```python
from build123d import *

# Parameters (mm, degrees)
F1_DEPTH = 9
F2_DEPTH = 1
F3_START = 8.8
F3_DEPTH = 0.2


with BuildPart() as f1:
    # F0 (on Top) → F1 (new body)
    with BuildSketch(Plane.XY):
        with BuildLine():
            Line((28.9218353152, 47.4191074908), (-98.2781646848, 47.4191074908))
            ThreePointArc((-98.2781646848, 47.4191074908), (-103.2279121531, 45.3688549591), (-105.2781646848, 40.4191074908))
            Line((-105.2781646848, 40.4191074908), (-105.2781646848, -18.9808925092))
            ThreePointArc((-105.2781646848, -18.9808925092), (-103.2279121531, -23.9306399775), (-98.2781646848, -25.9808925092))
            Line((-98.2781646848, -25.9808925092), (28.9218353152, -25.9808925092))
            ThreePointArc((28.9218353152, -25.9808925092), (33.8715827835, -23.9306399775), (35.9218353152, -18.9808925092))
            Line((35.9218353152, -18.9808925092), (35.9218353152, 40.4191074908))
            ThreePointArc((35.9218353152, 40.4191074908), (33.8715827835, 45.3688549591), (28.9218353152, 47.4191074908))
        make_face()
        with BuildLine():
            ThreePointArc((-104.7781646848, 39.9191074908), (-102.7279121531, 44.8688549591), (-97.7781646848, 46.9191074908))
            Line((-97.7781646848, 46.9191074908), (28.4218353152, 46.9191074908))
            ThreePointArc((28.4218353152, 46.9191074908), (33.3715827835, 44.8688549591), (35.4218353152, 39.9191074908))
            Line((35.4218353152, 39.9191074908), (35.4218353152, -18.4808925092))
            ThreePointArc((35.4218353152, -18.4808925092), (33.3715827835, -23.4306399775), (28.4218353152, -25.4808925092))
            Line((28.4218353152, -25.4808925092), (-97.7781646848, -25.4808925092))
            ThreePointArc((-97.7781646848, -25.4808925092), (-102.7279121531, -23.4306399775), (-104.7781646848, -18.4808925092))
            Line((-104.7781646848, -18.4808925092), (-104.7781646848, 10.7191074908))
            Line((-104.7781646848, 10.7191074908), (-104.7781646848, 39.9191074908))
        make_face(mode=Mode.SUBTRACT)
    extrude(amount=F1_DEPTH)

    # F0 (on Top) → F2 (join)
    with BuildSketch(Plane.XY):
        with BuildLine():
            Line((28.9218353152, 47.4191074908), (-98.2781646848, 47.4191074908))
            ThreePointArc((-98.2781646848, 47.4191074908), (-103.2279121531, 45.3688549591), (-105.2781646848, 40.4191074908))
            Line((-105.2781646848, 40.4191074908), (-105.2781646848, -18.9808925092))
            ThreePointArc((-105.2781646848, -18.9808925092), (-103.2279121531, -23.9306399775), (-98.2781646848, -25.9808925092))
            Line((-98.2781646848, -25.9808925092), (28.9218353152, -25.9808925092))
            ThreePointArc((28.9218353152, -25.9808925092), (33.8715827835, -23.9306399775), (35.9218353152, -18.9808925092))
            Line((35.9218353152, -18.9808925092), (35.9218353152, 40.4191074908))
            ThreePointArc((35.9218353152, 40.4191074908), (33.8715827835, 45.3688549591), (28.9218353152, 47.4191074908))
        make_face()
        with BuildLine():
            ThreePointArc((-104.7781646848, 39.9191074908), (-102.7279121531, 44.8688549591), (-97.7781646848, 46.9191074908))
            Line((-97.7781646848, 46.9191074908), (28.4218353152, 46.9191074908))
            ThreePointArc((28.4218353152, 46.9191074908), (33.3715827835, 44.8688549591), (35.4218353152, 39.9191074908))
            Line((35.4218353152, 39.9191074908), (35.4218353152, -18.4808925092))
            ThreePointArc((35.4218353152, -18.4808925092), (33.3715827835, -23.4306399775), (28.4218353152, -25.4808925092))
            Line((28.4218353152, -25.4808925092), (-97.7781646848, -25.4808925092))
            ThreePointArc((-97.7781646848, -25.4808925092), (-102.7279121531, -23.4306399775), (-104.7781646848, -18.4808925092))
            Line((-104.7781646848, -18.4808925092), (-104.7781646848, 10.7191074908))
            Line((-104.7781646848, 10.7191074908), (-104.7781646848, 39.9191074908))
        make_face(mode=Mode.SUBTRACT)
        with BuildLine():
            Line((28.4218353152, 46.9191074908), (-97.7781646848, 46.9191074908))
            ThreePointArc((-97.7781646848, 46.9191074908), (-102.7279121531, 44.8688549591), (-104.7781646848, 39.9191074908))
            Line((-104.7781646848, 39.9191074908), (-104.7781646848, 10.7191074908))
            Line((-104.7781646848, 10.7191074908), (-104.7781646848, -18.4808925092))
            ThreePointArc((-104.7781646848, -18.4808925092), (-102.7279121531, -23.4306399775), (-97.7781646848, -25.4808925092))
            Line((-97.7781646848, -25.4808925092), (28.4218353152, -25.4808925092))
            ThreePointArc((28.4218353152, -25.4808925092), (33.3715827835, -23.4306399775), (35.4218353152, -18.4808925092))
            Line((35.4218353152, -18.4808925092), (35.4218353152, 39.9191074908))
            ThreePointArc((35.4218353152, 39.9191074908), (33.3715827835, 44.8688549591), (28.4218353152, 46.9191074908))
        make_face()
        with BuildLine():
            Line((-104.0281646848, -17.7308925092), (-104.0281646848, 10.7191074908))
            Line((-104.0281646848, 10.7191074908), (-104.0281646848, 39.1691074908))
            ThreePointArc((-104.0281646848, 39.1691074908), (-101.9779121531, 44.1188549591), (-97.0281646848, 46.1691074908))
            Line((-97.0281646848, 46.1691074908), (27.6718353152, 46.1691074908))
            ThreePointArc((27.6718353152, 46.1691074908), (32.6215827835, 44.1188549591), (34.6718353152, 39.1691074908))
            Line((34.6718353152, 39.1691074908), (34.6718353152, -17.7308925092))
            ThreePointArc((34.6718353152, -17.7308925092), (32.6215827835, -22.6806399775), (27.6718353152, -24.7308925092))
            Line((27.6718353152, -24.7308925092), (-97.0281646848, -24.7308925092))
            ThreePointArc((-97.0281646848, -24.7308925092), (-101.9779121531, -22.6806399775), (-104.0281646848, -17.7308925092))
        make_face(mode=Mode.SUBTRACT)
        with BuildLine():
            Line((-104.0281646848, 39.1691074908), (-104.0281646848, 10.7191074908))
            Line((-104.0281646848, 10.7191074908), (-104.0281646848, -17.7308925092))
            ThreePointArc((-104.0281646848, -17.7308925092), (-101.9779121531, -22.6806399775), (-97.0281646848, -24.7308925092))
            Line((-97.0281646848, -24.7308925092), (27.6718353152, -24.7308925092))
            ThreePointArc((27.6718353152, -24.7308925092), (32.6215827835, -22.6806399775), (34.6718353152, -17.7308925092))
            Line((34.6718353152, -17.7308925092), (34.6718353152, 39.1691074908))
            ThreePointArc((34.6718353152, 39.1691074908), (32.6215827835, 44.1188549591), (27.6718353152, 46.1691074908))
            Line((27.6718353152, 46.1691074908), (-97.0281646848, 46.1691074908))
            ThreePointArc((-97.0281646848, 46.1691074908), (-101.9779121531, 44.1188549591), (-104.0281646848, 39.1691074908))
        make_face()
        with BuildLine():
            ThreePointArc((-68.7781646848, 10.7191074908), (-74.5312646848, 4.9660074908), (-80.2843646848, 10.7191074908))
            ThreePointArc((-80.2843646848, 10.7191074908), (-80.2676868415, 11.1568522219), (-80.2177500076, 11.5920589691))
            add(Edge.make_bspline(
                [(-80.2177500076, 11.5920589691), (-79.9166287785, 16.380589161), (-77.2316050473, 21.7170679747), (-74.5312646848, 21.7191074908)],
                knots=[0.0288652727, 0.0288652727, 0.0288652727, 0.0288652727, 0.4998199399, 0.4998199399, 0.4998199399, 0.4998199399], degree=3))
            add(Edge.make_bspline(
                [(-74.5312646848, 21.7191074908), (-71.6633529752, 21.7212735703), (-68.7781646848, 15.7063938677), (-68.7781646848, 10.7191074908)],
                knots=[0.4998199399, 0.4998199399, 0.4998199399, 0.4998199399, 1, 1, 1, 1], degree=3))
        make_face(mode=Mode.SUBTRACT)
        with BuildLine():
            ThreePointArc((28.3885360956, 14.3148952636), (28.6533737253, 14.9542698611), (29.2927483228, 15.2191074908))
            Line((29.2927483228, 15.2191074908), (30.4843238684, 15.2191074908))
            ThreePointArc((30.4843238684, 15.2191074908), (31.1236984659, 14.9542698611), (31.3885360956, 14.3148952636))
            Line((31.3885360956, 14.3148952636), (31.3885360956, 7.1233197179))
            ThreePointArc((31.3885360956, 7.1233197179), (31.1236984659, 6.4839451205), (30.4843238684, 6.2191074908))
            Line((30.4843238684, 6.2191074908), (29.2927483228, 6.2191074908))
            ThreePointArc((29.2927483228, 6.2191074908), (28.6533737253, 6.4839451205), (28.3885360956, 7.1233197179))
            Line((28.3885360956, 7.1233197179), (28.3885360956, 14.3148952636))
        make_face(mode=Mode.SUBTRACT)
    extrude(amount=F2_DEPTH)

    # F0 (on Top) → F3 (join)
    with BuildSketch(Plane.XY.offset(F3_START)):
        with BuildLine():
            Line((28.4218353152, 46.9191074908), (-97.7781646848, 46.9191074908))
            ThreePointArc((-97.7781646848, 46.9191074908), (-102.7279121531, 44.8688549591), (-104.7781646848, 39.9191074908))
            Line((-104.7781646848, 39.9191074908), (-104.7781646848, 10.7191074908))
            Line((-104.7781646848, 10.7191074908), (-104.7781646848, -18.4808925092))
            ThreePointArc((-104.7781646848, -18.4808925092), (-102.7279121531, -23.4306399775), (-97.7781646848, -25.4808925092))
            Line((-97.7781646848, -25.4808925092), (28.4218353152, -25.4808925092))
            ThreePointArc((28.4218353152, -25.4808925092), (33.3715827835, -23.4306399775), (35.4218353152, -18.4808925092))
            Line((35.4218353152, -18.4808925092), (35.4218353152, 39.9191074908))
            ThreePointArc((35.4218353152, 39.9191074908), (33.3715827835, 44.8688549591), (28.4218353152, 46.9191074908))
        make_face()
        with BuildLine():
            Line((-104.0281646848, -17.7308925092), (-104.0281646848, 10.7191074908))
            Line((-104.0281646848, 10.7191074908), (-104.0281646848, 39.1691074908))
            ThreePointArc((-104.0281646848, 39.1691074908), (-101.9779121531, 44.1188549591), (-97.0281646848, 46.1691074908))
            Line((-97.0281646848, 46.1691074908), (27.6718353152, 46.1691074908))
            ThreePointArc((27.6718353152, 46.1691074908), (32.6215827835, 44.1188549591), (34.6718353152, 39.1691074908))
            Line((34.6718353152, 39.1691074908), (34.6718353152, -17.7308925092))
            ThreePointArc((34.6718353152, -17.7308925092), (32.6215827835, -22.6806399775), (27.6718353152, -24.7308925092))
            Line((27.6718353152, -24.7308925092), (-97.0281646848, -24.7308925092))
            ThreePointArc((-97.0281646848, -24.7308925092), (-101.9779121531, -22.6806399775), (-104.0281646848, -17.7308925092))
        make_face(mode=Mode.SUBTRACT)
    extrude(amount=F3_DEPTH)


solid = f1.part
```
Design review of the part built by this model. Coordinates are the model's own, in mm. A direction names the side the tool comes from. Give positions to 0.01 mm unless a question says otherwise; leave off trailing zeros. Write each loop counter-clockwise with the first axis right and the second up, starting at its lowest first coordinate (ties: lowest second). Pieces come first, ordered by that corner, then holes. Notation, with made-up numbers: (51, -1) -> (73, -1) arc R18 ccw to (73, 30) -> close; hole circle Ø4 at (-33, 33). An arc over 180 degrees is marked (long way). Answer in a Markdown table with one row per item.
(1) Consider section C-C (y = 29.5). State the section outline as (x, z) points.
Results:
| item | result |
|---|---|
| outline | (-105.28, 0) -> (35.92, 0) -> (35.92, 9) -> (34.67, 9) -> (34.67, 8.8) -> (35.42, 8.8) -> (35.42, 1) -> (-104.78, 1) -> (-104.78, 8.8) -> (-104.03, 8.8) -> (-104.03, 9) -> (-105.28, 9) -> close |
(2) Consider section A-A (z = 5.75). State the section outline as (x, y) points, then the cut area to 3 significant figures.
Results:
| item | result |
|---|---|
| outline | (-105.28, -18.98) arc R7 ccw to (-98.28, -25.98) -> (28.92, -25.98) arc R7 ccw to (35.92, -18.98) -> (35.92, 40.42) arc R7 ccw to (28.92, 47.42) -> (-98.28, 47.42) arc R7 ccw to (-105.28, 40.42) -> close; hole (-104.78, -18.48) arc R7 ccw to (-97.78, -25.48) -> (28.42, -25.48) arc R7 ccw to (35.42, -18.48) -> (35.42, 39.92) arc R7 ccw to (28.42, 46.92) -> (-97.78, 46.92) arc R7 ccw to (-104.78, 39.92) -> close |
| area | 214 mm2 |
(3) Clearance check with flat-ended pins moving along their axes: pin 1 (12 mm diameter, centred on x = -68.5, y = 21.5, fed in from +Z); pin 2 (0.8 mm diameter, centred on x = 30, z = 0.5, fed in from +Y); pin 3 (1.1 mm diameter, centred on x = 30, z = 0.5, fed in from -Y). State where each tip first meets the part, or that it passes through.
Results:
| item | result |
|---|---|
| pin 1 | z = 1 |
| pin 2 | y = 47.39 |
| pin 3 | y = -25.96 |
(4) To check wall thickness, follow probe 1 along X at (y, z) = (-13.5, 2); probe 2 along Y at (x, z) = (-62, 4.5); probe 3 along X at (y, z) = (-21.5, 5.5). State the ranges of each line that lie inside material, in increasing order.
Results:
| item | result |
|---|---|
| probe 1 | -105.28 to -104.78, 35.42 to 35.92 |
| probe 2 | -25.98 to -25.48, 46.92 to 47.42 |
| probe 3 | -104.81 to -104.09, 34.74 to 35.45 |
(5) For faces 1 (the flat face through (-34, -25.481, 5)), 2 (the cylindrical face through (-103.28, -23.88, 4.44)), list the 3-axis set-ups (+Z, -Z, +X, -X, +Y, -Y) from which the entire face can be reached by the end or side of a thin tool; tool diameter is ignored.
Results:
| item | result |
|---|---|
| face 1 | none |
| face 2 | +Z, -Z, -X, -Y |
(6) Mouldability with a two-part tool opening along Y and no side actions: class faces 3 (the flat face through (-105.278, 11, 4)), 4 (the flat face through (-34, 47.419, 4)), 5 (the flat face through (35.422, 11, 5)) as +Y half, -Y half, draft (parallel to the pull), parting line (faces both ways), or undercut.
Results:
| item | result |
|---|---|
| face 3 | draft |
| face 4 | +Y half |
| face 5 | undercut |
(7) Consider section B-B (x = 15). State the section outline as (y, z) points, then the cut area to 3 significant figures.
Results:
| item | result |
|---|---|
| outline | (-25.98, 0) -> (47.42, 0) -> (47.42, 9) -> (46.17, 9) -> (46.17, 8.8) -> (46.92, 8.8) -> (46.92, 1) -> (-25.48, 1) -> (-25.48, 8.8) -> (-24.73, 8.8) -> (-24.73, 9) -> (-25.98, 9) -> close |
| area | 81.7 mm2 |
